Autodesk Inventor part; units mm, degrees
ref_plane "YZ Plane" through (0, 0, 0) normal (1, 0, 0) x (0, 1, 0)
ref_plane "XZ Plane" through (0, 0, 0) normal (0, 1, 0) x (-1, 0, 0)
ref_plane "XY Plane" through (0, 0, 0) normal (0, 0, 1) x (1, 0, 0)
sketch "Sketch1" plane through (0, 0, 0) normal (0, 0, 1) x (1, 0, 0)
  line L0 (12, 17.5) -> (-13, 17.5)
  line L1 (-13, 17.5) -> (-13, -17.5)
  line L2 (-13, -17.5) -> (12, -17.5)
  line L3 (12, -17.5) -> (12, 17.5)
  point P0 (0, 0)
  point P1 (12, 0)
  dimension "d0" = 25
  dimension "d1" = 35
  dimension "d16" = 12
extrude "Extrusion1" add sketch "Sketch1" along normal blind 5
sketch "Sketch2" plane through (0, 0, 5) normal (0, 0, 1) x (1, 0, 0)
  circle A0 centre (0, 0) radius 3.05
  dimension "d4" = 6.1
extrude "Extrusion2" cut sketch "Sketch2" against normal up to next
sketch "Sketch4" plane through (0, 0, 5) normal (0, 0, 1) x (1, 0, 0)
  circle A0 centre (0, 0) radius 3.05
  arc A1 (-7, -3.0859) -> (-5.7899, 5) centre (0, 0) ccw
  line L0 (-5.7899, 5) -> (-11, 5)
  line L1 (-11, 5) -> (-11, -17.5)
  line L2 (-13, -17.5) -> (12, -17.5)
  line L3 (-7, -3.0859) -> (-7, -17.5)
  circle A2 centre (0, 0) radius 3.05
  line L4 (12, 17.5) -> (-13, 17.5)
  line L5 (-13, 17.5) -> (-13, -17.5)
  line L6 (-13, -17.5) -> (12, -17.5)
  line L7 (12, -17.5) -> (12, 17.5)
  dimension "d9" = 15.3
  dimension "d10" = 11
  dimension "d11" = 7
  dimension "d12" = 5
extrude "Extrusion3" add sketch "Sketch4" along normal blind 15 contours A1 L0 L1 L2 L5 L4 L7 L3
fillet "Fillet1" radius 2 3 edges at (-7, -3.0859, 12.5) (-5.7899, 5, 12.5) (-11, 5, 12.5)
sketch "Sketch5" plane through (0, 0, 20) normal (0, 0, 1) x (1, 0, 0)
  point P0 (0, 0)
  point P1 (-8, 12)
  point P2 (7, -12)
  dimension "d17" = 7
  dimension "d18" = 12
  dimension "d19" = 12
  dimension "d20" = 8
hole "Hole1" at (-8, 12, 20) at (7, -12, 20) direction (0, 0, -1) diameter 4.2 depth 8 tip angle 118 countersink diameter 6 countersink angle 90
chamfer "Chamfer1" distance 1 angle 45 6 edges at (7.606, 0.819, 20) (-5.9817, -6.5111, 20) (-7, -12.8768, 20) (-5.9014, 5.1424, 20) (-7.8212, 5, 20) (-11, -7.25, 20)
properties part number "Base" material "ABS Plastic"
Can you work these out from the model? Positions are in its coordinate system, mm. A direction names the side the tool comes from. Round coordinates to 2 decimals unless told otherwise and drop trailing zeros. Write each loop counter-clockwise with the first axis right and the second up, starting at its lowest first coordinate (ties: lowest second). Pieces come first, ordered by that corner, then holes. Notation, with made-up numbers: (-27.75, 62.25) - (22.25, 62.25) arc R19 cw to (22.25, 73.25) - close; hole circle Ø3 at (28.5, 87.5). An arc over 180 degrees is marked (long way). Write each question's results on one line, items separated by ' | '. Start each with the question number.
1) Suppose I cut it at B-B (z = 14.25). List the corners of the cut face in (x, y) for me, and give its area (3 significant figures).
2) Which directions (+Z, -Z, +X, -X, +Y, -Y) give clear straight access to the entire face, cutting with the end or side of a thin tool? Please do faces 1 (the cylindrical face through (7.577, 1.055, 11.902)), 2 (the flat face through (-11.5, -7.4, 19.5)), 3 (the flat face through (-3.5, 0.2, 0)).
3) Suppose I cut it at A-A (z = 3). List the corners of the cut face in (x, y) for me.
4) We'd pull the mould along X, two halves only. Please class faces 4 (the flat face through (-7.8, 5.5, 19.5)), 5 (the flat face through (12, 0, 10)), 6 (the flat face through (-13, 0, 10)), 7 (the cylindrical face through (-3.047, 0.134, 2.535)): released by +X, released by -X, zero draft, split by the parting line, or undercut.
5) Please list where these lines run through material, in increasing order: line 1 (Y direction, x = 0, z = 2.95); line 2 (X direction, y = 12, z = 14.75); line 3 (Y direction, x = -8, z = 17.5).
6) For pin 1 Ø2.5 at (x, y) = (-8, 12) entering from +Z, with a flat end and sliding along its axis, tell me the tip position at first contact or that it passes through.
Here are the results:
1) outline: (-13, -17.5) - (-11, -17.5) - (-11, 3) arc R2 cw to (-9, 5) - (-6.64, 5) arc R2 ccw to (-5.27, 5.55) arc R7.65 cw (long way) to (-3.96, -6.54) arc R2 ccw to (-7, -8.25) - (-7, -17.5) - (12, -17.5) - (12, 17.5) - (-13, 17.5) - close; hole circle Ø4.2 at (-8, 12); hole circle Ø4.2 at (7, -12) | area: 572 mm2
2) face 1: +Z | face 2: +Z, -Y | face 3: -Z, +X, -X, +Y, -Y
3) outline: (-13, -17.5) - (12, -17.5) - (12, 17.5) - (-13, 17.5) - close; hole circle Ø6.1 at (0, 0)
4) face 4: undercut | face 5: released by +X | face 6: released by -X | face 7: undercut
5) line 1: y = -17.5 to -3.05, 3.05 to 17.5 | line 2: x = -13 to -10.1, -5.9 to 12 | line 3: y = 5 to 9.9, 14.1 to 17.5
6) pin 1: stops at z = 11.49
